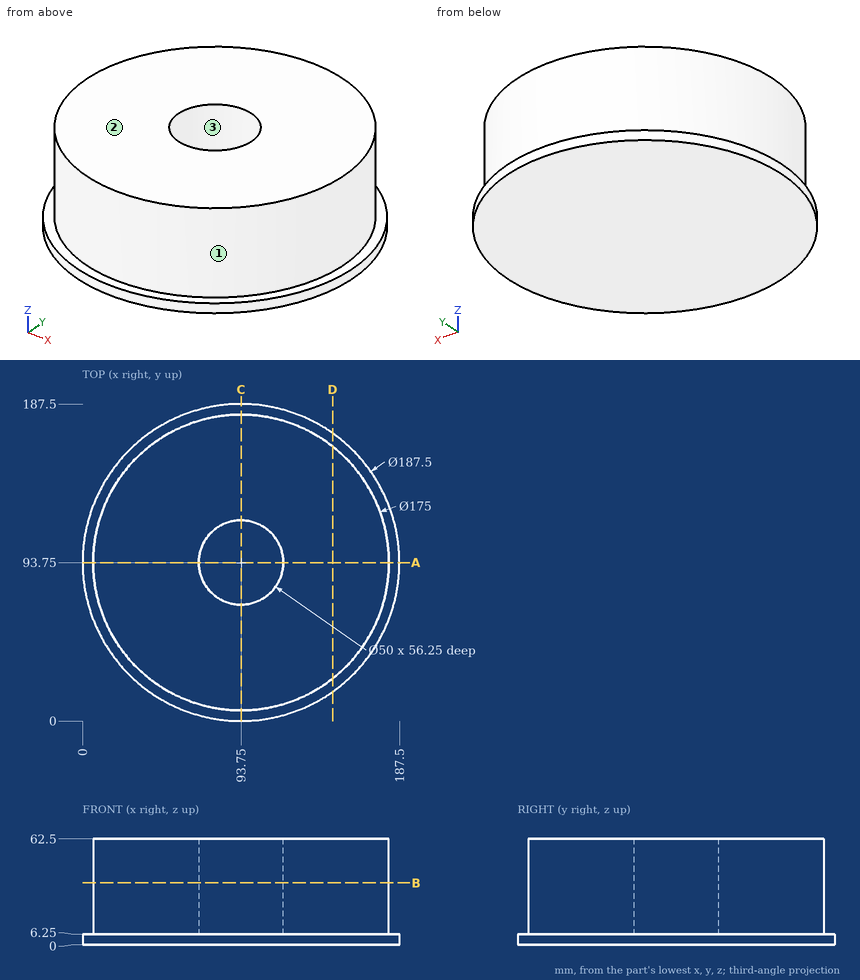
Here's the drawing with two shaded views (mm, measured from the low corner). I have some questions. Give positions to 0.01 mm unless a question says otherwise; leave off trailing zeros. Write each loop counter-clockwise with the first axis right and the second up, starting at its lowest first coordinate (ties: lowest second). Pieces come first, ordered by that corner, then holes. Notation, with made-up numbers: (59, 70.25) -> (76, 70.25) arc R19 ccw to (76, 76.25) -> close; hole circle Ø2 at (47.25, -27.75). An arc over 180 degrees is marked (long way). Answer as a JSON object with one key per item and string values. Group by question number.
Item 1: Suppose I cut it at D-D (x = 148). Please give me the cut outline in (y, z), plus the area to 3 significant figures.
Item 2: Suppose I cut it at A-A (y = 93.75). Please give me the cut outline in (x, z).
Item 3: I'm going to push flat-ended pins straight in: P1, Ø8, axis at x = 131.5, z = 10.5, coming from the +Y side; P2, Ø6, axis at x = 167, z = 43, coming from the -Y side (3 decimals); P3, Ø4, axis at y = 55.5, z = 8, coming from the -X side; P4, Ø12, axis at y = 92, z = 9.5, coming from the +X side. Where does each tip first touch, or does it pass through?
Item 4: Suppose I cut it at B-B (z = 36.5). Please give me the cut outline in (x, y).
Item 5: Please list where these lines run through material, in increasing order: line 1 (X direction, y = 93.75, z = 34); line 2 (Y direction, x = 93, z = 36); line 3 (Y direction, x = 94, z = 4). Write a range as [from, to].
Item 6: We'd pull the mould along X, two halves only. Please class the marked faces 1, 2 and 3: +X half, -X half, draft (parallel to the pull), parting line (faces both ways), or undercut.
Findings:
{
 "1": {"outline": "(17.29, 0) -> (170.21, 0) -> (170.21, 6.25) -> (162.4, 6.25) -> (162.4, 62.5) -> (25.1, 62.5) -> (25.1, 6.25) -> (17.29, 6.25) -> close", "area": "8,680 mm²"},
 "2": {"outline": "(0, 0) -> (187.5, 0) -> (187.5, 6.25) -> (181.25, 6.25) -> (181.25, 62.5) -> (118.75, 62.5) -> (118.75, 6.25) -> (68.75, 6.25) -> (68.75, 62.5) -> (6.25, 62.5) -> (6.25, 6.25) -> (0, 6.25) -> close"},
 "3": {"P1": "stops at y = 174.48", "P2": "stops at y = 41.585", "P3": "stops at x = 7.73", "P4": "stops at x = 187.5"},
 "4": {"outline": "circle Ø175 at (93.75, 93.75); hole circle Ø50 at (93.75, 93.75)"},
 "5": {"line 1": "x = [6.25, 68.75], [118.75, 181.25]", "line 2": "y = [6.25, 68.76], [118.74, 181.25]", "line 3": "y = [0, 187.5]"},
 "6": {"face 1": "parting line", "face 2": "draft", "face 3": "undercut"}
}
